Build history of the part. All positions in model axes, mm. A direction names the side the tool comes from. Give positions to 0.01 mm unless a question says otherwise; leave off trailing zeros. Order: outer loops, then holes, each group sorted by start corner. A loop starts at its lowest first (then second) coordinate and runs counter-clockwise, first axis right, second up. Notation, with made-up numbers: (-2.5, 14) -> (34.5, 14) arc R19 ccw to (34.5, 35) -> close; hole circle Ø8 at (-3.5, 82). An arc over 180 degrees is marked (long way). One line per question, with ' | ' between items. Start each with the question number.
(1) Cut at B-B (x = 81). Give the cut face in (y, z), then the cut area to 3 significant figures.
(2) Pin check, flat tips, straight feed: pin 1 Ø10 at (x, z) = (4, -20.5) entering from +Y; pin 2 Ø8 at (x, z) = (147.5, 31.5) entering from +Y. Stop position of each tip, or through.
(3) Which spindle directions (+Z, -Z, +X, -X, +Y, -Y) get a long thin tool onto all of the face, cutting with end or side? Do faces 1 (the face through (62, 63.4, 44.5)), 2 (the face through (6, 243.7, 1)), 3 (the face through (0, 124, 1)), 4 (the face through (12.7, 127, 1)), 5 (the face through (192, 6, -50.8)). Say none if no direction does.
(4) Cut at C-C (z = -31). Give the cut face in (x, y), then the cut area to 3 significant figures.
(5) Cut at A-A (y = 99). Give the cut face in (x, z).
(6) Pull direction X, two halves, no side cores. Call faces 6 (the face through (192, 6, 50.8)), 7 (the face through (195, 12.7, 1)), 8 (the face through (62, 63.4, -44.5)), 9 (the face through (385.8, 148, 1)): +X half, -X half, draft (parallel to the pull), parting line (faces both ways), or undercut.
(7) Drill centre lines: L1, parallel to X at y = 166.5, z = 6; L2, parallel to Z at x = 58, y = 29; L3, parallel to Y at x = 284.5, z = 28. Where is each one in solid material? Low to high. Write a range as from..to.
(8) Cut at D-D (y = 201). Give the cut face in (x, z), then the cut area to 3 significant figures.
from build123d import *

# Parameters (mm, degrees)
BOSS_EXTRUDE1_DEPTH = 50.8
BOSS_EXTRUDE2_DEPTH = 12.7


with BuildPart() as part:
    # Sketch1 → Boss-Extrude1 (new, symmetric)
    with BuildSketch(Plane.XY):
        Polygon((0, 0), (385.8, 0), (385.8, 300), (373.1, 300), (373.1, 12.7), (12.7, 12.7), (12.7, 243.7), (0, 243.7), (0, 12.7), align=None)
    extrude(amount=BOSS_EXTRUDE1_DEPTH, both=True)

    # Sketch2 → Boss-Extrude2 (add)
    with BuildSketch(Plane.XY.offset(50.8)):
        Polygon((373.1, 112.7), (273.1, 12.7), (373.1, 12.7), align=None)
        Polygon((12.7, 12.7), (12.7, 112.7), (112.7, 12.7), align=None)
    boss_extrude2 = extrude(amount=-BOSS_EXTRUDE2_DEPTH)

    # Mirror1: Boss-Extrude2 across plane
    add(boss_extrude2.mirror(Plane.XY))


solid = part.part
Result set:
1) outline: (0, -50.8) -> (44.4, -50.8) -> (44.4, -38.1) -> (12.7, -38.1) -> (12.7, 38.1) -> (44.4, 38.1) -> (44.4, 50.8) -> (0, 50.8) -> close | area: 2,100 mm2
2) pin 1: stops at y = 243.7 | pin 2: stops at y = 12.7
3) face 1: +Z, -Z, +Y | face 2: +Z, -Z, -X, +Y | face 3: +Z, -Z, -X, +Y, -Y | face 4: +Y | face 5: -Z, +X, -X, +Y, -Y
4) outline: (0, 0) -> (385.8, 0) -> (385.8, 300) -> (373.1, 300) -> (373.1, 12.7) -> (12.7, 12.7) -> (12.7, 243.7) -> (0, 243.7) -> close | area: 11,500 mm2
5) outline: (0, -50.8) -> (26.4, -50.8) -> (26.4, -38.1) -> (12.7, -38.1) -> (12.7, 38.1) -> (26.4, 38.1) -> (26.4, 50.8) -> (0, 50.8) -> close; (359.4, -50.8) -> (385.8, -50.8) -> (385.8, 50.8) -> (359.4, 50.8) -> (359.4, 38.1) -> (373.1, 38.1) -> (373.1, -38.1) -> (359.4, -38.1) -> close
6) face 6: draft | face 7: undercut | face 8: undercut | face 9: +X half
7) L1: x = 0..12.7, 373.1..385.8 | L2: z = -50.8..-38.1, 38.1..50.8 | L3: y = 0..12.7
8) outline: (0, -50.8) -> (12.7, -50.8) -> (12.7, 50.8) -> (0, 50.8) -> close; (373.1, -50.8) -> (385.8, -50.8) -> (385.8, 50.8) -> (373.1, 50.8) -> close | area: 2,580 mm2
